Model file for the job. Use its own axes, mm. A direction names the side the tool comes from. Round coordinates to 2 decimals unless told otherwise and drop trailing zeros. Order: outer loops, then holes, each group sorted by start corner. A loop starts at its lowest first (then second) coordinate and runs counter-clockwise, first axis right, second up. Notation, with made-up numbers: (80.25, 76.25) -> (129.25, 76.25) arc R27 ccw to (129.25, 95.25) -> close; hole circle Ø5 at (52.25, 1). An arc over 180 degrees is marked (long way). Answer as CSV lines item,"result".
Autodesk Inventor part; units mm, degrees
ref_plane "YZ Plane" through (0, 0, 0) normal (1, 0, 0) x (0, 1, 0)
ref_plane "XZ Plane" through (0, 0, 0) normal (0, 1, 0) x (-1, 0, 0)
ref_plane "XY Plane" through (0, 0, 0) normal (0, 0, 1) x (1, 0, 0)
sketch "Sketch1" plane through (0, 0, 0) normal (0, 0, 1) x (1, 0, 0)
  line L0 (0, 0) -> (22.352, 0)
  line L1 (22.352, 0) -> (22.352, 12.7)
  line L2 (22.352, 12.7) -> (0, 12.7)
  line L3 (0, 12.7) -> (0, 0)
  dimension "d0" = 22.352
  dimension "d1" = 12.7
extrude "Extrusion1" add sketch "Sketch1" against normal blind 1.5875
sketch "Sketch2" plane through (0, 0, 0) normal (0, 0, 1) x (1, 0, 0)
  line L0 (22.352, 0) -> (22.352, 12.7)
  line L1 (6.6675, 14.9342) -> (15.6845, 14.9342)
  line L2 (15.6845, 14.9342) -> (15.6845, 7.3142)
  line L3 (15.6845, 7.3142) -> (6.6675, 7.3142)
  line L4 (6.6675, 7.3142) -> (6.6675, 14.9342)
  dimension "d8" = 9.017
  dimension "d9" = 7.62
  dimension "d10" = 6.6675
extrude "Extrusion2" add sketch "Sketch2" along normal blind 3.175
fillet "Fillet1" radius 1.5875 4 edges at (15.6845, 11.1242, 3.175) (15.6845, 13.8171, 0) (6.6675, 11.1242, 3.175) (6.6675, 13.8171, 0)
properties part number "‎BOB-15100‎ USB C Breakout" material "PBT Plastic"
Q1. Saw through at A-A (y = 8.5). Write the cut outline in (x, z) (1 decimal), plus the area to 3 significant figures.
Checks:
outline,"(0, -1.6) -> (22.4, -1.6) -> (22.4, 0) -> (15.7, 0) -> (15.7, 1.6) arc R1.6 ccw to (14.1, 3.2) -> (8.3, 3.2) arc R1.6 ccw to (6.7, 1.6) -> (6.7, 0) -> (0, 0) -> close"
area,"63.0 mm²"
Q2. Saw through at C-C (z = 0.95). Write the cut outline in (x, y), plus the area to 3 significant figures.
Checks:
outline,"(6.67, 7.31) -> (15.68, 7.31) -> (15.68, 12.7) -> (15.55, 12.7) -> (15.55, 14.93) -> (6.8, 14.93) -> (6.8, 12.7) -> (6.67, 12.7) -> close"
area,"68.1 mm²"
Q3. Wall check: L1, parallel to X at y = 11.75, z = 1.2; L2, parallel to Y at x = 14.5, z = 1.3; L3, parallel to Y at x = 12.5, z = -0.25. Give the ranges that are in metal, low to high. Write a range as [from, to].
Checks:
L1,"[6.67, 15.68]"
L2,"[7.31, 14.93]"
L3,"[0, 12.7]"
Q4. Saw through at B-B (x = 10). Write the cut outline in (y, z) (1 decimal), plus the area to 3 significant figures.
Checks:
outline,"(0, -1.6) -> (12.7, -1.6) -> (12.7, 0) -> (14.9, 0) -> (14.9, 3.2) -> (7.3, 3.2) -> (7.3, 0) -> (0, 0) -> close"
area,"44.4 mm²"
Q5. Tool access for faces 1 (the flat face through (11, 14, 0)), 2 (the flat face through (11, 7.314, 2)), 3 (the cylindrical face through (15.207, 13.801, 0.453)), 4 (the flat face through (6.668, 9, 1)), 5 (the flat face through (15.684, 10, 1)): list every direction of +Z, -Z, +X, -X, +Y, -Y with a clear straight run to the whole face (end or side of a thin tool).
Checks:
face 1,"-Z, +X, -X, +Y"
face 2,"+Z, +X, -X, -Y"
face 3,"-Z, +X, +Y"
face 4,"+Z, -X, +Y, -Y"
face 5,"+Z, +X, +Y, -Y"
Q6. Flat gauge pins, fed straight in: pin 1 (1.7 mm diameter, centred on y = 10.5, z = 1, fed in from +X); pin 2 (2 mm diameter, centred on y = 3.5, z = 1.5, fed in from +X) (1 decimal); pin 3 (1.5 mm diameter, centred on x = 6, z = 0.5, fed in from +Y); pin 4 (1 mm diameter, centred on x = 13, z = 1.5, fed in from -Y). Where does each tip first touch, or does it go through?
Checks:
pin 1,"x = 15.68"
pin 2,"through"
pin 3,"y = 12.7"
pin 4,"y = 7.31"
Q7. Saw through at D-D (x = 20.5). Write the cut outline in (y, z).
Checks:
outline,"(0, -1.59) -> (12.7, -1.59) -> (12.7, 0) -> (0, 0) -> close"
